```python
from build123d import *

# Parameters (mm, degrees)
BOSS_EXTRUDE1_DEPTH      = 22
SKETCH3_R                = 1.55
CUT_EXTRUDE1_DEPTH       = 30
CUT_EXTRUDE5_DEPTH       = 9
SKETCH11_R               = 0.75
CUT_EXTRUDE10_DEPTH      = 13
CUT_EXTRUDE11_START      = -10
CUT_EXTRUDE11_DEPTH      = 10
SKETCH13_R               = 3
SKETCH13_R_2             = 1.5
CUT_EXTRUDE12_DEPTH      = 4
FILLET1_SIZE             = 7
SKETCH14_W               = 54
SKETCH14_H               = 9.3
SKETCH14_W_2             = 7.05
SKETCH14_H_2             = 4
BOSS_EXTRUDE4_DEPTH      = 4
SKETCH17_W               = 7.05
SKETCH17_H               = 4
BOSS_EXTRUDE5_DEPTH      = 23.05
BOSS_EXTRUDE6_DEPTH      = 27.3
BOSS_EXTRUDE6_DEPTH_BACK = 4
SKETCH18_W               = 54
SKETCH18_H               = 2.95
SKETCH19_W               = 54
SKETCH19_H               = 2.8
BOSS_EXTRUDE7_DEPTH      = 21
FILLET2_SIZE             = 6.5
FILLET3_SIZE             = 0.5
SKETCH20_R               = 3.970030919
BOSS_EXTRUDE8_DEPTH      = 6
FILLET4_R                = 1
CUT_EXTRUDE13_START      = -37.3
CUT_EXTRUDE13_DEPTH      = 37.3
SKETCH22_W               = 56.118071471
SKETCH22_H               = 11.813110758
CUT_EXTRUDE14_DEPTH      = 56
BOSS_EXTRUDE9_DEPTH      = 4
BOSS_EXTRUDE9_DEPTH_BACK = 26
SKETCH23_W               = 67
SKETCH23_H               = 4
SKETCH25_W               = 5
SKETCH25_H               = 30
BOSS_EXTRUDE10_DEPTH     = 7.07
SKETCH26_W               = 5
SKETCH26_H               = 5
BOSS_EXTRUDE11_DEPTH     = 7.07
SKETCH27_R               = 1.5
CUT_EXTRUDE15_DEPTH      = 7.07
SKETCH28_W               = 5
SKETCH28_H               = 20
SKETCH28_W_2             = 15
CUT_EXTRUDE16_DEPTH      = 7.07
SKETCH29_W               = 3.5
SKETCH29_H               = 30
BOSS_EXTRUDE12_DEPTH     = 47
SKETCH31_W               = 3.5
SKETCH31_H               = 2
CUT_EXTRUDE18_DEPTH      = 47
FILLET8_R                = 3
SKETCH34_W               = 47
SKETCH34_H               = 2.99
BOSS_EXTRUDE14_DEPTH     = 23.3
CUT_EXTRUDE19_DEPTH      = 38
CUT_EXTRUDE20_DEPTH      = 7.07
SKETCH37_R               = 2.5
BOSS_EXTRUDE15_DEPTH     = 7
FILLET10_R               = 0.5


# Read off the part's stored shape, not the designer's step: Cut-Extrude13
with BuildPart() as part:
    # Sketch1 → Boss-Extrude1 (new body)
    with BuildSketch(Plane(origin=(0, 0, 0), x_dir=(1, 0, 0), z_dir=(0, 1, 0))):
        Polygon((0, 0), (0, 50), (67, 50), (67, 0), (63, 0), (63, 46), (4, 46), (4, 0), align=None)
    extrude(amount=BOSS_EXTRUDE1_DEPTH)

    # Sketch3 → Cut-Extrude1 (cut)
    with BuildSketch(Plane(origin=(67, 0, 0), x_dir=(0, 0, -1), z_dir=(1, 0, 0))):
        with Locations((12.05, 11)):
            Circle(SKETCH3_R)
    extrude(amount=-CUT_EXTRUDE1_DEPTH, mode=Mode.SUBTRACT)

    # Sketch5 → Cut-Extrude5 (cut)
    with BuildSketch(Plane(origin=(67, 0, 0), x_dir=(0, 0, -1), z_dir=(1, 0, 0))):
        with BuildLine():
            Line((12.05, 22), (0, 22))
            Line((0, 22), (0, 0))
            Line((0, 0), (12.05, 0))
            ThreePointArc((12.05, 0), (1.05, 11), (12.05, 22))
        make_face()
    extrude(amount=-CUT_EXTRUDE5_DEPTH, mode=Mode.SUBTRACT)

    # Sketch11 → Cut-Extrude10 (cut)
    with BuildSketch(Plane(origin=(67, 0, 0), x_dir=(0, 0, -1), z_dir=(1, 0, 0))):
        with Locations((19.05, 11)):
            Circle(SKETCH11_R)
        with Locations((12.05, 18)):
            Circle(SKETCH11_R)
        with Locations((12.05, 4)):
            Circle(SKETCH11_R)
        with Locations((5.05, 11)):
            Circle(SKETCH11_R)
    extrude(amount=-CUT_EXTRUDE10_DEPTH, mode=Mode.SUBTRACT)

    # Sketch12 → Cut-Extrude11 (cut)
    with BuildSketch(Plane.ZY.offset(CUT_EXTRUDE11_START)):
        with BuildLine():
            Line((-12.05, 22), (0, 22))
            Line((0, 22), (0, 0))
            Line((0, 0), (-12.05, 0))
            ThreePointArc((-12.05, 0), (-1.05, 11), (-12.05, 22))
        make_face()
    extrude(amount=CUT_EXTRUDE11_DEPTH, mode=Mode.SUBTRACT)

    # Sketch13 → Cut-Extrude12 (cut)
    with BuildSketch(Plane.ZY):
        with Locations((-12.05, 11)):
            Circle(SKETCH13_R)
        with Locations((-19.05, 11)):
            Circle(SKETCH13_R_2)
        with Locations((-12.05, 4)):
            Circle(SKETCH13_R_2)
        with Locations((-5.05, 11)):
            Circle(SKETCH13_R_2)
        with Locations((-12.05, 18)):
            Circle(SKETCH13_R_2)
    extrude(amount=-CUT_EXTRUDE12_DEPTH, mode=Mode.SUBTRACT)

    # Fillet1
    fillet1_edges = [part.edges().sort_by_distance(p)[0] for p in [
        (63, 11, -46),
        (4, 11, -46),
    ]]
    chamfer(fillet1_edges, length=FILLET1_SIZE)

    # Sketch14 → Boss-Extrude4 (add)
    with BuildSketch(Plane(origin=(0, 0, -50), x_dir=(-1, 0, 0), z_dir=(0, 0, -1))):
        with Locations((-33.5, -4.65)):
            Rectangle(SKETCH14_W, SKETCH14_H)
        with Locations((-56.975, 20)):
            Rectangle(SKETCH14_W_2, SKETCH14_H_2)
        with Locations((-10.025, 20)):
            Rectangle(SKETCH14_W_2, SKETCH14_H_2)
    extrude(amount=-BOSS_EXTRUDE4_DEPTH)

    # Sketch17 → Boss-Extrude5 (add)
    with BuildSketch(Plane(origin=(0, 0, -50), x_dir=(-1, 0, 0), z_dir=(0, 0, -1))):
        with Locations((-56.975, 20)):
            Rectangle(SKETCH17_W, SKETCH17_H)
        with Locations((-10.025, 20)):
            Rectangle(SKETCH17_W, SKETCH17_H)
    extrude(amount=BOSS_EXTRUDE5_DEPTH)

    # Sketch18 → Boss-Extrude6 (add, two sides: drawn at the far end of the back side and taken through both)
    with BuildSketch(Plane.XZ.offset(-18).offset(-BOSS_EXTRUDE6_DEPTH_BACK)):
        with Locations((33.5, -71.575)):
            Rectangle(SKETCH18_W, SKETCH18_H)
    extrude(amount=BOSS_EXTRUDE6_DEPTH + BOSS_EXTRUDE6_DEPTH_BACK)

    # Sketch19 → Boss-Extrude7 (add)
    with BuildSketch(Plane(origin=(0, 0, -50), x_dir=(-1, 0, 0), z_dir=(0, 0, -1))):
        with Locations((-33.5, -7.9)):
            Rectangle(SKETCH19_W, SKETCH19_H)
    extrude(amount=BOSS_EXTRUDE7_DEPTH)

    # Fillet2
    fillet2_edges = [part.edges().sort_by_distance(p)[0] for p in [
        (60.5, 20, -50),
        (6.5, 20, -50),
    ]]
    chamfer(fillet2_edges, length=FILLET2_SIZE - 0.0001)  # a hair under: the kernel refuses the full size

    # Fillet3
    fillet3_edges = [part.edges().sort_by_distance(p)[0] for p in [
        (60.5, 6.35, -73.05),
        (6.5, 6.35, -73.05),
    ]]
    chamfer(fillet3_edges, length=FILLET3_SIZE)

    # Sketch20 → Boss-Extrude8 (add)
    with BuildSketch(Plane.XZ.offset(9.3)):
        with Locations(Location((23.4, -59.65, 0), (0, 0, 270))):
            Circle(SKETCH20_R)
    extrude(amount=BOSS_EXTRUDE8_DEPTH)

    # Fillet4
    fillet4_edges = [part.edges().sort_by_distance(p)[0] for p in [
        (23.4, -15.3, -55.679969081),
    ]]
    fillet(fillet4_edges, radius=FILLET4_R)

    # Cut-Extrude13 outline → Cut-Extrude13 (cut)
    with BuildSketch(Plane(origin=(0, 22, 0), x_dir=(1, 0, 0), z_dir=(0, 1, 0)).offset(CUT_EXTRUDE13_START)):
        Polygon((67, 50), (60.5, 56.5), (60.5, 72.55), (60, 73.05), (7, 73.05), (6.5, 72.55), (6.5, 56.5), (0, 50), align=None)
    extrude(amount=CUT_EXTRUDE13_DEPTH, mode=Mode.SUBTRACT)

    # Sketch22 → Cut-Extrude14 (cut)
    with BuildSketch(Plane(origin=(0, 0, -50), x_dir=(-1, 0, 0), z_dir=(0, 0, -1))):
        with Locations((-32.440964265, -5.906555379)):
            Rectangle(SKETCH22_W, SKETCH22_H)
    extrude(amount=-CUT_EXTRUDE14_DEPTH, mode=Mode.SUBTRACT)

    # Sketch23 → Boss-Extrude9 (add, two sides: drawn at the far end of the back side and taken through both)
    with BuildSketch(Plane(origin=(0, 22, 0), x_dir=(1, 0, 0), z_dir=(0, 1, 0)).offset(-BOSS_EXTRUDE9_DEPTH_BACK)):
        with Locations((33.5, 48)):
            Rectangle(SKETCH23_W, SKETCH23_H)
    extrude(amount=BOSS_EXTRUDE9_DEPTH + BOSS_EXTRUDE9_DEPTH_BACK)

    # Sketch25 → Boss-Extrude10 (add)
    with BuildSketch(Plane(origin=(0, 0, -50), x_dir=(-1, 0, 0), z_dir=(0, 0, -1))):
        with Locations((-41.9, 11)):
            Rectangle(SKETCH25_W, SKETCH25_H)
    extrude(amount=BOSS_EXTRUDE10_DEPTH)

    # Sketch26 → Boss-Extrude11 (add)
    with BuildSketch(Plane(origin=(0, 0, -50), x_dir=(-1, 0, 0), z_dir=(0, 0, -1))):
        with Locations((-46.9, 23.5)):
            Rectangle(SKETCH26_W, SKETCH26_H)
        with Locations((-46.9, -1.5)):
            Rectangle(SKETCH26_W, SKETCH26_H)
    extrude(amount=BOSS_EXTRUDE11_DEPTH)

    # Sketch27 → Cut-Extrude15 (cut)
    with BuildSketch(Plane(origin=(44.4, 0, 0), x_dir=(0, 0, -1), z_dir=(1, 0, 0))):
        with Locations((52.3, 6)):
            Circle(SKETCH27_R)
        with Locations((52.3, 16.11)):
            Circle(SKETCH27_R)
    extrude(amount=-CUT_EXTRUDE15_DEPTH, mode=Mode.SUBTRACT)

    # Sketch28 → Cut-Extrude16 (cut)
    with BuildSketch(Plane(origin=(0, 0, -50), x_dir=(-1, 0, 0), z_dir=(0, 0, -1))):
        with Locations((-46.9, 11)):
            Rectangle(SKETCH28_W, SKETCH28_H)
        with Locations((-31.9, 11)):
            Rectangle(SKETCH28_W_2, SKETCH28_H)
    extrude(amount=-CUT_EXTRUDE16_DEPTH, mode=Mode.SUBTRACT)

    # Sketch29 → Boss-Extrude12 (add)
    with BuildSketch(Plane(origin=(0, 0, -50), x_dir=(-1, 0, 0), z_dir=(0, 0, -1))):
        with Locations((-14.35, 11)):
            Rectangle(SKETCH29_W, SKETCH29_H)
    extrude(amount=BOSS_EXTRUDE12_DEPTH)

    # Sketch31 → Cut-Extrude18 (cut)
    with BuildSketch(Plane(origin=(0, 0, -97), x_dir=(-1, 0, 0), z_dir=(0, 0, -1))):
        with Locations((-14.35, 25)):
            Rectangle(SKETCH31_W, SKETCH31_H)
        with Locations((-14.35, -3)):
            Rectangle(SKETCH31_W, SKETCH31_H)
    extrude(amount=-CUT_EXTRUDE18_DEPTH, mode=Mode.SUBTRACT)

    # Fillet8
    fillet8_edges = [part.edges().sort_by_distance(p)[0] for p in [
        (39.4, 1, -48),
        (39.4, 21, -48),
        (24.4, 21, -48),
        (24.4, 1, -48),
    ]]
    fillet(fillet8_edges, radius=FILLET8_R)

    # Sketch34 → Boss-Extrude14 (add)
    with BuildSketch(Plane(origin=(16.1, 0, 0), x_dir=(0, 0, -1), z_dir=(1, 0, 0))):
        with Locations((73.5, 22.505)):
            Rectangle(SKETCH34_W, SKETCH34_H)
        with Locations((73.5, -0.505)):
            Rectangle(SKETCH34_W, SKETCH34_H)
    extrude(amount=BOSS_EXTRUDE14_DEPTH)

    # Sketch35 → Cut-Extrude19 (cut)
    with BuildSketch(Plane.XZ.offset(2)):
        Polygon((39.4, -57.07), (17.6, -97), (39.4, -97), align=None)
    extrude(amount=-CUT_EXTRUDE19_DEPTH, mode=Mode.SUBTRACT)

    # Sketch36 → Cut-Extrude20 (cut)
    with BuildSketch(Plane(origin=(0, 0, -57.07), x_dir=(-1, 0, 0), z_dir=(0, 0, -1))):
        Polygon((-39.4, 24), (-41.4, 26), (-39.4, 26), align=None)
        Polygon((-39.4, -2), (-39.4, -4), (-41.4, -4), align=None)
    extrude(amount=-CUT_EXTRUDE20_DEPTH, mode=Mode.SUBTRACT)

    # Sketch37 → Boss-Extrude15 (add)
    with BuildSketch(Plane.ZY.offset(-12.6)):
        with Locations(Location((-87.1, 11, 0), (0, 0, 90))):
            Circle(SKETCH37_R)
    extrude(amount=BOSS_EXTRUDE15_DEPTH)

    # Fillet10
    fillet10_edges = [part.edges().sort_by_distance(p)[0] for p in [
        (5.6, 8.5, -87.1),
    ]]
    fillet(fillet10_edges, radius=FILLET10_R)


solid = part.part
```
Could you check a few things on this model? Use its own coordinates, in mm. A direction names the side the tool comes from. Round coordinates to 2 decimals unless told otherwise and drop trailing zeros. Loops run counter-clockwise (first coordinate to the right, second up) from the corner with the lowest first, then second, coordinate; pieces in that order, holes last. Notation, with made-up numbers: (-15.5, 36) - (9.5, 36) arc R5 ccw to (9.5, 42) - close; hole circle Ø4 at (37, -26). An arc over 180 degrees is marked (long way). Use CSV: the item, a comma, the result in double quotes.
Item 1: If we section it at C-C on z = -87.1: List the corners of the cut face in (x, y) for me, then the cut area to 3 significant figures.
Here are the results:
outline,"(5.6, 9) arc R0.5 ccw to (6.1, 8.5) - (12.6, 8.5) - (12.6, -2) - (23, -2) - (23, 0.99) - (16.1, 0.99) - (16.1, 21.01) - (23, 21.01) - (23, 24) - (12.6, 24) - (12.6, 13.5) - (6.1, 13.5) arc R0.5 ccw to (5.6, 13) - close"
area,"167 mm²"
Item 2: If we mould it in two halves opening along X, with no side actions, what happens to faces 1 (the flat face through (32, 21, -48)), 2 (the flat face through (40.4, 25, -53.6)), 3 (the flat face through (64, 0, -33)), 4 (the flat face through (39.4, 11, -51))? For each: pulls with the +X half, pulls with the -X half, needs draft (parallel to the pull), parting line crosses it, or undercut.
Here are the results:
face 1,"undercut"
face 2,"pulls with the -X half"
face 3,"needs draft"
face 4,"undercut"
Item 3: For faces 5 (the flat face through (8, 11, -43)), 6 (the flat face through (49.4, 11, -48)), 7 (the cylindrical face through (9.4, 10.67, -89.58)), 8 (the flat face through (22, 11, -50)), 9 (the flat face through (64, 22, -33)), which set-ups out of +Z, -Z, +X, -X, +Y, -Y let a thin tool reach every point of the face, with its end or its side?
Here are the results:
face 5,"+Z, +Y, -Y"
face 6,"+Z, -Z"
face 7,"-X"
face 8,"-Z"
face 9,"+Z, +X, -X, +Y"
Item 4: Will these pins go through, and if not, where does the flat tip stop? pin 1 (5 mm diameter, centred on x = 51, y = 9.5, fed in from -Z); pin 2 (21.5 mm diameter, centred on x = 30, z = -68, fed in from +Y); pin 3 (1 mm diameter, centred on y = 14.5, z = -83.5, fed in from +X).
Here are the results:
pin 1,"stops at z = -50"
pin 2,"stops at y = 24"
pin 3,"stops at x = 16.1"
Item 5: If we section it at B-B on z = -25: List the corners of the cut face in (x, y) for me.
Here are the results:
outline,"(0, 0) - (4, 0) - (4, 22) - (0, 22) - close; (63, 0) - (67, 0) - (67, 22) - (63, 22) - close"
Item 6: If we section it at A-A on z = -52.3: List the corners of the cut face in (x, y) for me.
Here are the results:
outline,"(12.6, -2) - (39.4, -2) - (41.4, -4) - (49.4, -4) - (49.4, 1) - (44.4, 1) - (44.4, 4.5) - (39.4, 4.5) - (39.4, 0.99) - (16.1, 0.99) - (16.1, 21.01) - (39.4, 21.01) - (39.4, 17.61) - (44.4, 17.61) - (44.4, 21) - (49.4, 21) - (49.4, 26) - (41.4, 26) - (39.4, 24) - (12.6, 24) - close; (39.4, 7.5) - (44.4, 7.5) - (44.4, 14.61) - (39.4, 14.61) - close"
Item 7: I need wall thicknesses on L1, parallel to Y at x = 63.9, z = -12.05; L2, parallel to X at y = 8, z = -6; L3, parallel to Y at x = 22.5, z = -76.5. Which ranges of each line are inside material? Lowest first, please. Write a range as [from, to].
Here are the results:
L1,"y = [0, 3.25], [4.75, 9.45], [12.55, 17.25], [18.75, 22]"
L2,"x = [0, 4], [63, 67]"
L3,"y = [-2, 0.99], [21.01, 24]"
